```python
from build123d import *

# Parameters (mm, degrees)
SKETCH1_W           = 150
SKETCH1_H           = 150
BOSS_EXTRUDE1_DEPTH = 30
SKETCH2_R           = 50
BOSS_EXTRUDE2_DEPTH = 1
SKETCH3_W           = 25
SKETCH3_H           = 30
SKETCH3_W_2         = 30
SKETCH3_H_2         = 25
BOSS_EXTRUDE3_DEPTH = 1.25
SCALE1_SCALE        = 0.5


with BuildPart() as part:
    # Sketch1 → Boss-Extrude1 (new body, symmetric)
    with BuildSketch(Plane.XY):
        Rectangle(SKETCH1_W, SKETCH1_H)
    extrude(amount=BOSS_EXTRUDE1_DEPTH, both=True)

    # Sketch2 → Boss-Extrude2 (add)
    with BuildSketch(Plane.XY.offset(30)):
        Circle(SKETCH2_R)
    extrude(amount=BOSS_EXTRUDE2_DEPTH)

    # Sketch3 → Boss-Extrude3 (add)
    with BuildSketch(Plane.XY.offset(30)):
        with Locations((-27.5, 0)):
            Rectangle(SKETCH3_W, SKETCH3_H)
        Rectangle(SKETCH3_W_2, SKETCH3_H)
        with Locations((0, 27.5)):
            Rectangle(SKETCH3_W_2, SKETCH3_H_2)
        with Locations((27.5, 0)):
            Rectangle(SKETCH3_W, SKETCH3_H)
        with Locations((0, -27.5)):
            Rectangle(SKETCH3_W_2, SKETCH3_H_2)
    extrude(amount=BOSS_EXTRUDE3_DEPTH)


with BuildPart() as part_1:
    # Scale1: scaled about (0, 0, 0.198621989)
    add(part.part.scale(SCALE1_SCALE).moved(Location((0, 0, 0.099310994))))


solid = part_1.part
```
Geometry check sheet. Reference: the model listing, model coordinates, mm. A direction names the side the tool comes from. Round coordinates to 2 decimals unless told otherwise and drop trailing zeros. Loops run counter-clockwise (first coordinate to the right, second up) from the corner with the lowest first, then second, coordinate; pieces in that order, holes last. Notation, with made-up numbers: (80, 84) - (85, 84) arc R23 cw to (85, 103) - close; hole circle Ø5 at (39, 63). An arc over 180 degrees is marked (long way). Write item = value, one per line. Start each with the question number.
1. Depth check by flat-ended pin: pin 1 (6 mm diameter, centred on x = 6, y = 26, fed in from +Z); pin 2 (3 mm diameter, centred on x = -26.5, y = 2.5, fed in from +Z). Enter the tip coordinate at first touch or a pass-through.
2. Set-up check for faces 1 (the face through (23.846, 7.509, 15.346)), 2 (the face through (0, 0, 15.724)): record each of +Z, -Z, +X, -X, +Y, -Y from which the full face is reachable in a straight line by a thin tool's end or side.
3. Section check A-A on y = -33. Enter the section's corners in (x, z), then the cut area to 3 significant figures.
4. Thickness scan on line 1 (Z direction, x = 8.5, y = 14.5); line 2 (Z direction, x = 25, y = -8). Record the ranges inside material, lowest first.
Working result:
q1.pin_1 = 15.6
q1.pin_2 = 15.1
q2.face_1 = +Z
q2.face_2 = +Z, +X, -X, +Y, -Y
q3.outline = (-37.5, -14.9) - (37.5, -14.9) - (37.5, 15.1) - (-37.5, 15.1) - close
q3.area = 2,250 mm^2
q4.line_1 = -14.9 to 15.6
q4.line_2 = -14.9 to 15.1
